Autodesk Inventor part; units mm, degrees
ref_plane "YZ Plane" through (0, 0, 0) normal (1, 0, 0) x (0, 1, 0)
ref_plane "XZ Plane" through (0, 0, 0) normal (0, 1, 0) x (-1, 0, 0)
ref_plane "XY Plane" through (0, 0, 0) normal (0, 0, 1) x (1, 0, 0)
sketch "Sketch1" plane through (0, 0, 0) normal (0, 0, 1) x (1, 0, 0)
  line L0 (0, 0) -> (50, 0)
  line L1 (50, 0) -> (50, 25)
  line L2 (50, 25) -> (0, 25)
  line L3 (0, 25) -> (0, 0)
  line L4 (47, 3) -> (3, 3)
  line L5 (3, 3) -> (3, 22)
  line L6 (3, 22) -> (47, 22)
  line L7 (47, 22) -> (47, 3)
  dimension "d0" = 50
  dimension "d1" = 25
  dimension "d2" = 3
extrude "Extrusion1" add sketch "Sketch1" along normal blind 600
sketch "Sketch2" plane through (0, 25, 0) normal (0, 1, 0) x (1, 0, 0)
  line L0 (50, -600) -> (0, -600)
  point P0 (0, 0)
  point P1 (25, -562.5)
  point P2 (25, -37.5)
  dimension "d5" = 37.5
  dimension "d6" = 37.5
  dimension "d7" = 25
hole "Hole1" at (25, 25, 562.5) at (25, 25, 37.5) direction (0, -1, 0) diameter 6 end through all counterbore diameter 11 counterbore depth 5
sketch "Sketch4" plane through (50, 0, 0) normal (1, 0, 0) x (0, 0, -1)
  line L0 (0, 0) -> (66.9632, 0)
  point P0 (-100, 12.5)
  point P1 (-200, 12.5)
  point P2 (-300, 12.5)
  point P3 (-400, 12.5)
  point P4 (-500, 12.5)
  dimension "d31" = 100
  dimension "d32" = 12.5
  dimension "d36" = 100
hole "Hole3" at (50, 12.5, 100) at (50, 12.5, 200) at (50, 12.5, 300) at (50, 12.5, 400) at (50, 12.5, 500) direction (-1, 0, 0) diameter 5 depth 8 tip angle 118
sketch "Sketch6" plane through (0, 25, 0) normal (0, 1, 0) x (1, 0, 0)
  line L0 (50, -600) -> (0, -600)
  point P0 (0, 0)
  point P1 (29, -239)
  point P2 (29, -361)
  dimension "d60" = 239
  dimension "d61" = 29
  dimension "d69" = 239
hole "Hole5" at (29, 25, 239) at (29, 25, 361) direction (0, -1, 0) diameter 28.575 end through all
sketch "Sketch7" plane through (0, 0, 0) normal (0, 1, 0) x (1, 0, 0)
  line L0 (50, 0) -> (50, -600)
  line L1 (50, 0) -> (0, 0)
  point P0 (41, -330)
  point P1 (9, -330)
  point P2 (9, -270)
  point P3 (41, -270)
  dimension "d70" = 9
  dimension "d71" = 9
  dimension "d72" = 60
  dimension "d73" = 600
  dimension "d74" = 270
hole "Hole6" at (41, 0, 330) at (9, 0, 330) at (9, 0, 270) at (41, 0, 270) direction (0, 1, 0) diameter 5 depth 8
properties part number "Back Bar"
Work out the finished part from the listing and answer in its coordinate system (mm). A direction names the side the tool comes from. Coordinates: 2 decimals unless noted, no trailing zeros. Loops run counter-clockwise (first coordinate to the right, second up) from the corner with the lowest first, then second, coordinate; pieces in that order, holes last.
1) Flat-ended cylindrical pins translate along their axes: pin 1 (3 mm diameter, centred on y = 12.5, z = 100, fed in from +X); pin 2 (10 mm diameter, centred on x = 25, z = 37.5, fed in from +Y). Find the tip coordinate at first contact, or state that the pin passes through.
Results:
pin 1: stops at x = 3
pin 2: stops at y = 3
2) Section B-B (z = 130.5) is taken. Give the vertices of the cut face in (x, y).
Results:
outline: (0, 0) - (50, 0) - (50, 25) - (0, 25) - close; hole (3, 3) - (47, 3) - (47, 22) - (3, 22) - close
3) Section A-A (z = 239) is taken. Give the vertices of the cut face in (x, y).
Results:
outline: (0, 0) - (14.71, 0) - (14.71, 3) - (3, 3) - (3, 22) - (14.71, 22) - (14.71, 25) - (0, 25) - close; (43.29, 0) - (50, 0) - (50, 25) - (43.29, 25) - (43.29, 22) - (47, 22) - (47, 3) - (43.29, 3) - close
4) For a pull along Z with two mould halves and no side action, classify faces 1 (the flat face through (25, 23, 0)), 2 (the flat face through (47, 13, 296)), 3 (the cylindrical face through (28.372, 1.479, 224.726)) as +Z half, -Z half, draft (parallel to the pull), parting line (faces both ways), or undercut.
Results:
face 1: -Z half
face 2: draft
face 3: undercut
5) Section C-C (z = 366) is taken. Give the vertices of the cut face in (x, y), plus the area to 3 significant figures.
Results:
outline: (0, 0) - (15.62, 0) - (15.62, 3) - (3, 3) - (3, 22) - (15.62, 22) - (15.62, 25) - (0, 25) - close; (42.38, 0) - (50, 0) - (50, 25) - (42.38, 25) - (42.38, 22) - (47, 22) - (47, 3) - (42.38, 3) - close
area: 253 mm2
6) For faces 4 (the cylindrical face through (23.348, 23.479, 567.746)), 5 (the flat face through (25, 0, 296)), 6 (the flat face through (25, 22, 296)), determine the directions among +Z, -Z, +X, -X, +Y, -Y from which every point of the face is accessible in a straight line to the end or side of a thin tool.
Results:
face 4: +Y
face 5: +Z, -Z, +X, -X, -Y
face 6: +Z, -Z
7) Consider probe 1 along Z at (x, y) = (9, 1); probe 2 along Z at (x, y) = (48.05, 12.5); probe 3 along Z at (x, y) = (29, 1.05). Determine where each line is inside the solid, lowest interval first.
Results:
probe 1: z = 0 to 267.5, 272.5 to 327.5, 332.5 to 600
probe 2: z = 0 to 97.5, 102.5 to 197.5, 202.5 to 297.5, 302.5 to 397.5, 402.5 to 497.5, 502.5 to 600
probe 3: z = 0 to 224.71, 253.29 to 346.71, 375.29 to 600
